Design review of the part built by this model. Coordinates are the model's own, in mm. A direction names the side the tool comes from. Coordinates: 2 decimals unless noted, no trailing zeros. Order: outer loops, then holes, each group sorted by start corner. A loop starts at its lowest first (then second) coordinate and runs counter-clockwise, first axis right, second up. Notation, with made-up numbers: (44.5, 27.5) -> (92.5, 27.5) arc R33 ccw to (92.5, 65.5) -> close; hole circle Ø3 at (63, 47). An arc over 180 degrees is marked (long way). Write item = value, one per line.
```python
from build123d import *

# Parameters (mm, degrees)
F3_DEPTH = 8


# Not quite as in the source:
# - after a boolean that leaves OpenCascade's solid faulty, fix() repairs it


with BuildPart() as f1:
    # F0 (on Front) → F1 (revolve)
    with BuildSketch(Plane.XZ):
        Polygon((2.5, 5), (0, 5), (0, -25), (3.5, -25), (3.5, 0), (7.5, 0), (7.5, 17), (2.5, 17), align=None)
    revolve(axis=Axis((0, 0, -10), (0, 0, -1)))

    # F2 (on face) → F3 (join)
    with BuildSketch(Plane.XY.offset(17)):
        with BuildLine():
            ThreePointArc((7.5, 0), (5.5789784011, 5.0124844139), (0.8, 7.457211275))
            Line((0.8, 7.457211275), (0.8, 2.3685438565))
            ThreePointArc((0.8, 2.3685438565), (2.0310096012, 1.4577379737), (2.5, 0))
            ThreePointArc((2.5, 0), (2.466917068, -0.4053642552), (2.3685438565, -0.8))
            Line((2.3685438565, -0.8), (7.457211275, -0.8))
            ThreePointArc((7.457211275, -0.8), (7.4892951792, -0.4005717398), (7.5, 0))
        make_face()
        with BuildLine():
            Line((-2.3685438565, 0.8), (-7.457211275, 0.8))
            ThreePointArc((-7.457211275, 0.8), (-5.8387300862, -4.7073592363), (-0.8, -7.457211275))
            Line((-0.8, -7.457211275), (-0.8, -2.3685438565))
            ThreePointArc((-0.8, -2.3685438565), (-2.2404988474, -1.1091279975), (-2.3685438565, 0.8))
        make_face()
    extrude(amount=F3_DEPTH)

    add(f1.part.fix(), mode=Mode.REPLACE)


solid = f1.part
```
(1) For faces 1 (the flat face through (-2, 4, 17)), 2 (the flat face through (0.8, 5, 21)), 3 (the flat face through (3, -4, 17)), 4 (the flat face through (-3.2, -1.8, 0)), list the 3-axis set-ups (+Z, -Z, +X, -X, +Y, -Y) from which the entire face can be reached by the end or side of a thin tool; tool diameter is ignored.
Report:
face_1 = +Z, -X, +Y
face_2 = +Z, -X, +Y, -Y
face_3 = +Z, +X, -Y
face_4 = -Z
(2) We need section D-D (z = 13.5). Write out the cut boundary in (x, y), and give its area (3 significant figures).
Report:
outline = circle Ø15 at (0, 0); hole circle Ø5 at (0, 0)
area = 157 mm²
(3) We need section B-B (y = 4.5). Write out the cut boundary in (x, z), and give its area (3 significant figures).
Report:
outline = (-6, 0) -> (6, 0) -> (6, 25) -> (0.8, 25) -> (0.8, 17) -> (-6, 17) -> close
area = 246 mm²
(4) For L1, parallel to Y at x = 0, z = 11; L2, parallel to Z at x = 4.25, y = -4.75, list the stretches that pass through material, from the lowest coordinate up.
Report:
L1 = -7.5 to -2.5, 2.5 to 7.5
L2 = 0 to 17
(5) We need section A-A (z = 20.5). Write out the cut boundary in (x, y).
Report:
outline = (-7.46, 0.8) arc R7.5 ccw to (-0.8, -7.46) -> (-0.8, -2.37) arc R2.5 cw to (-2.37, 0.8) -> close; (0.8, 2.37) arc R2.5 cw to (2.37, -0.8) -> (7.46, -0.8) arc R7.5 ccw to (0.8, 7.46) -> close
(6) The part is to be moulded in two halves that separate along X. For faces 5 (the cylindrical face through (3.233, 1.341, -12.325)), 6 (the flat face through (-0.8, -5, 21)), 7 (the flat face through (-4, -3, 25)), 8 (the flat face through (0, 0, 5)), say which applies: released by +X, released by -X, zero draft, split by the parting line, or undercut.
Report:
face_5 = split by the parting line
face_6 = released by +X
face_7 = zero draft
face_8 = undercut
(7) We need section C-C (x = 0). Write out the cut boundary in (y, z), and give its area (3 significant figures).
Report:
outline = (-7.5, 0) -> (-3.5, 0) -> (-3.5, -25) -> (3.5, -25) -> (3.5, 0) -> (7.5, 0) -> (7.5, 17) -> (2.5, 17) -> (2.5, 5) -> (-2.5, 5) -> (-2.5, 17) -> (-7.5, 17) -> close
area = 370 mm²
(8) Insertion check: pin 1 (1.5 mm diameter, centred on x = 4.5, z = 21, fed in from -Y); pin 2 (3 mm diameter, centred on y = -3.5, z = -2.5, fed in from +X); pin 3 (1.5 mm diameter, centred on x = -0.5, z = 13, fed in from -Y); pin 4 (5.5 mm diameter, centred on y = -3.5, z = 20.5, fed in from +X). Each pin has a flat end and moves straight along its axis. Give the tip position at first contact, or say it passes through.
Report:
pin_1 = -0.8
pin_2 = 2.87
pin_3 = -7.5
pin_4 = 7.46
